Verification items for the finished model (mm, model axes). Coordinates: 2 decimals unless noted, no trailing zeros. Loops run counter-clockwise (first coordinate to the right, second up) from the corner with the lowest first, then second, coordinate; pieces in that order, holes last. Notation, with made-up numbers: (76.25, -0.75) - (129.25, -0.75) arc R23 ccw to (129.25, 13.25) - close; hole circle Ø6 at (83.5, 69.25). An arc over 180 degrees is marked (long way). One line per item, written item: value. Start each with the question number.
(1) Section check D-D (z = 3.5). Record the boundary of the cut face in (x, y), plus the area to 3 significant figures.
(2) Thickness scan on probe 1 along Z at (x, y) = (2.45, 7.62); probe 2 along Y at (x, z) = (2, 1.25); probe 3 along Y at (x, z) = (3.3, 0). Record the ranges inside material, lowest first. Write a range as [from, to].
(3) Section check A-A (z = 0). Record the boundary of the cut face in (x, y).
(4) Gauge pin test, flat ends, axial feed: P1, Ø1.5, axis at x = 0, z = 1, coming from the +Y side; P2, Ø1.5, axis at x = -3, y = 8.5, coming from the -Z side; P3, Ø3, axis at x = -2, z = 1.5, coming from the +Y side. Record the tip position at first contact, or that the pin passes through.
(5) Section check C-C (y = 7.62). Record the boundary of the cut face in (x, z) (1 decimal).
(6) Section check B-B (x = 2). Record the boundary of the cut face in (y, z) (1 decimal), plus the area to 3 significant figures.
```python
from build123d import *

# Parameters (mm, degrees)
SKETCH1_R               = 4.7625
BOSS_EXTRUDE1_DEPTH     = 17.78
CUT_EXTRUDE1_DEPTH      = 17.78
CUT_EXTRUDE1_DEPTH_BACK = 17.78
CUT_EXTRUDE2_DEPTH      = 17.78
CUT_EXTRUDE2_DEPTH_BACK = 17.78
SKETCH4_R               = 1.5875
CUT_EXTRUDE3_DEPTH      = 17.78
CUT_EXTRUDE3_DEPTH_BACK = 17.78


with BuildPart() as part:
    # Sketch1 → Boss-Extrude1 (new body)
    with BuildSketch(Plane(origin=(0, 0, 0), x_dir=(1, 0, 0), z_dir=(0, 1, 0))):
        Circle(SKETCH1_R)
    extrude(amount=BOSS_EXTRUDE1_DEPTH)

    # Sketch2 → Cut-Extrude1 (cut, two sides)
    with BuildSketch(Plane.XY) as cut_extrude1_sk:
        Polygon((-4.7625, 17.78), (0, 17.78), (-4.7625, 11.43), align=None)
    extrude(amount=CUT_EXTRUDE1_DEPTH, mode=Mode.SUBTRACT)
    extrude(cut_extrude1_sk.sketch, amount=-CUT_EXTRUDE1_DEPTH_BACK, mode=Mode.SUBTRACT)

    # Sketch3 → Cut-Extrude2 (cut, two sides)
    with BuildSketch(Plane.XY) as cut_extrude2_sk:
        Polygon((0, 17.78), (4.7625, 17.78), (4.7625, 11.43), align=None)
    extrude(amount=CUT_EXTRUDE2_DEPTH, mode=Mode.SUBTRACT)
    extrude(cut_extrude2_sk.sketch, amount=-CUT_EXTRUDE2_DEPTH_BACK, mode=Mode.SUBTRACT)

    # Sketch4 → Cut-Extrude3 (cut, two sides)
    with BuildSketch(Plane(origin=(0, 0, 0), x_dir=(0, 0, -1), z_dir=(1, 0, 0))) as cut_extrude3_sk:
        with Locations((0, 7.62)):
            Circle(SKETCH4_R)
    extrude(amount=CUT_EXTRUDE3_DEPTH, mode=Mode.SUBTRACT)
    extrude(cut_extrude3_sk.sketch, amount=-CUT_EXTRUDE3_DEPTH_BACK, mode=Mode.SUBTRACT)


solid = part.part
```
Responses:
1. outline: (-3.23, 0) - (3.23, 0) - (3.23, 13.47) - (0, 17.78) - (-3.23, 13.47) - close
1. area: 101 mm²
2. probe 1: z = [-4.08, -1.59], [1.59, 4.08]
2. probe 2: y = [0, 6.64], [8.6, 15.11]
2. probe 3: y = [0, 6.03], [9.21, 13.38]
3. outline: (-4.76, 0) - (4.76, 0) - (4.76, 6.03) - (-4.76, 6.03) - close; (-4.76, 9.21) - (4.76, 9.21) - (4.76, 11.43) - (0, 17.78) - (-4.76, 11.43) - close
4. P1: stops at y = 17.78
4. P2: stops at z = -4.2
4. P3: stops at y = 17.11
5. outline: (-4.5, -1.6) arc R4.8 ccw to (4.5, -1.6) - close; (-4.5, 1.6) - (4.5, 1.6) arc R4.8 ccw to start
6. outline: (0, -4.3) - (15.1, -4.3) - (15.1, 4.3) - (0, 4.3) - close; hole circle Ø3.2 at (7.6, 0)
6. area: 123 mm²
